Autodesk Inventor part; units mm, degrees
ref_plane "YZ Plane" through (0, 0, 0) normal (1, 0, 0) x (0, 1, 0)
ref_plane "XZ Plane" through (0, 0, 0) normal (0, 1, 0) x (-1, 0, 0)
ref_plane "XY Plane" through (0, 0, 0) normal (0, 0, 1) x (1, 0, 0)
sketch "Sketch1" plane through (0, 0, 0) normal (0, 1, 0) x (-1, 0, 0)
  circle A0 centre (0, 0) radius 4.9
  circle A1 centre (0, 0) radius 6.9
  line L0 (6.9, 8) -> (-5.9499, 8) construction
  line L1 (6.9, -8) -> (-5.9499, -8) construction
  line L2 (8, 8.15) -> (-8, 8.15)
  line L3 (-8, 8.15) -> (-8, -8.15)
  line L4 (-8, -8.15) -> (8, -8.15)
  line L5 (8, -8.15) -> (8, 8.15)
  line L6 (8, 8.15) -> (8, 10.15)
  line L7 (8, 10.15) -> (-8, 10.15)
  line L8 (-8, 10.15) -> (-8, 8.15)
  line L9 (-8, -8.15) -> (-8, -10.15)
  line L10 (-8, -10.15) -> (8, -10.15)
  line L11 (8, -10.15) -> (8, -8.15)
  point P0 (0, -8.15)
  dimension "d0" = 9.8
  dimension "d1" = 2
  dimension "d2" = 16
  dimension "d3" = 8
  dimension "d4" = 0.15
  dimension "d5" = 0.15
  dimension "d6" = 16
  dimension "d7" = 2
  dimension "d8" = 2
extrude "Extrusion1" add sketch "Sketch1" along normal blind 3 contours A1 | L5 L4 L3 L2 | L2 L8 L7 L6 | L11 L10 L9 L4
extrude "Extrusion2" add sketch "Sketch1" against normal blind 15 contours L2 L8 L7 L6 | L11 L10 L9 L4
sketch "Sketch2" plane through (-8, 3, 10.15) normal (0, 0, 1) x (1, 0, 0)
  circle A0 centre (8, -15) radius 1.65
  line L0 (16, -18) -> (0, -18)
  point P0 (8, -3)
  point P1 (8, -18)
  dimension "d13" = 3.3
  dimension "d14" = 3
extrude "Extrusion3" cut sketch "Sketch2" against normal through all
sketch "Sketch3" plane through (-8, 3, 10.15) normal (0, 0, 1) x (1, 0, 0)
  line L0 (8, -10) -> (8, -6) construction
  line L1 (9.65, -10) -> (9.65, -6)
  line L2 (6.35, -6) -> (6.35, -10)
  arc A0 (6.35, -10) -> (9.65, -10) centre (8, -10) ccw
  arc A1 (9.65, -6) -> (6.35, -6) centre (8, -6) ccw
  circle A2 centre (8, -15) radius 1.65
  point P0 (8, -3)
  point P1 (8, -8)
  dimension "d17" = 3.3
  dimension "d18" = 4
  dimension "d19" = 5
extrude "Extrusion4" cut sketch "Sketch3" against normal through all contours A0 L2 A1 L1
properties part number "ShaftSyncAdapter" material "ABS Plastic"
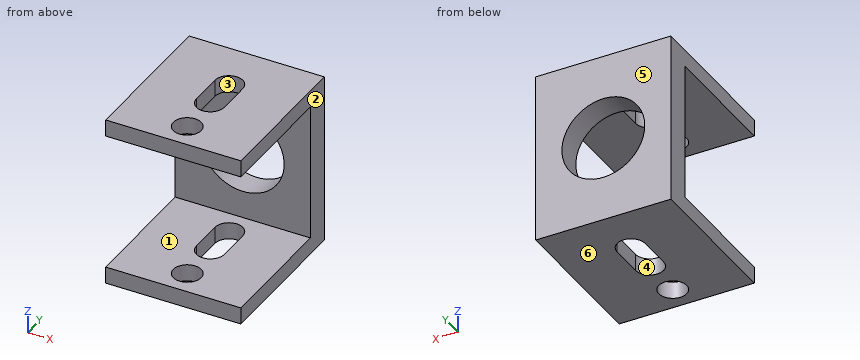
CAD build for the part. Positions are in the model's coordinates, mm. Face numbers are marked on the shaded views. A direction names the side the tool comes from. Give positions to 0.01 mm unless a question says otherwise; leave off trailing zeros. Write each loop counter-clockwise with the first axis right and the second up, starting at its lowest first coordinate (ties: lowest second). Pieces come first, ordered by that corner, then holes. Notation, with made-up numbers: (25, -23.5) - (54, -23.5) arc R21 cw to (54, -8.5) - close; hole circle Ø2 at (25, 56). An arc over 180 degrees is marked (long way). Put each result on its own line as item: value.
(1) Wall check: L1, parallel to Y at x = 0, z = 8.85; L2, parallel to Z at x = -6.75, y = -9.5; L3, parallel to Z at x = 0, y = 0.9. Give the ranges that are in metal, low to high.
Working result:
L1: -15 to -13.65, -10.35 to -8.65, -1.35 to 3
L2: -10.15 to -8.15, 8.15 to 10.15
L3: -10.15 to -4.9, 4.9 to 10.15
(2) Saw through at B-B (x = 0). List the corners of the cut face in (y, z).
Working result:
outline: (-15, -10.15) - (-13.65, -10.15) - (-13.65, -8.15) - (-15, -8.15) - close; (-15, 8.15) - (-13.65, 8.15) - (-13.65, 10.15) - (-15, 10.15) - close; (-10.35, -10.15) - (-8.65, -10.15) - (-8.65, -8.15) - (-10.35, -8.15) - close; (-10.35, 8.15) - (-8.65, 8.15) - (-8.65, 10.15) - (-10.35, 10.15) - close; (-1.35, -10.15) - (3, -10.15) - (3, -4.9) - (0, -4.9) - (0, -8.15) - (-1.35, -8.15) - close; (-1.35, 8.15) - (0, 8.15) - (0, 4.9) - (3, 4.9) - (3, 10.15) - (-1.35, 10.15) - close
(3) Tool access for the marked faces 1, 2 and 3: list every direction of +Z, -Z, +X, -X, +Y, -Y with a clear straight run to the whole face (end or side of a thin tool).
Working result:
face 1: +X, -X, -Y
face 2: +Z, -Z, +X, +Y, -Y
face 3: +Z, -Z
(4) Drop a flat-ended pin along its axis: pin 1 Ø8 at (x, z) = (1, 3.5) entering from -Y. Give the stop position or say it passes through.
Working result:
pin 1: y = 0
(5) Saw through at D-D (x = -2.75). List the corners of the cut face in (y, z).
Working result:
outline: (-15, -10.15) - (3, -10.15) - (3, -4.06) - (0, -4.06) - (0, -8.15) - (-15, -8.15) - close; (-15, 8.15) - (0, 8.15) - (0, 4.06) - (3, 4.06) - (3, 10.15) - (-15, 10.15) - close
(6) Saw through at A-A (y = -12). List the corners of the cut face in (x, z), then the cut area to 3 significant figures.
Working result:
outline: (-8, -10.15) - (-1.65, -10.15) - (-1.65, -8.15) - (-8, -8.15) - close; (-8, 8.15) - (-1.65, 8.15) - (-1.65, 10.15) - (-8, 10.15) - close; (1.65, -10.15) - (8, -10.15) - (8, -8.15) - (1.65, -8.15) - close; (1.65, 8.15) - (8, 8.15) - (8, 10.15) - (1.65, 10.15) - close
area: 50.8 mm^2
(7) Saw through at C-C (z = 0). List the corners of the cut face in (x, y).
Working result:
outline: (-8, 0) - (-4.9, 0) - (-4.9, 3) - (-8, 3) - close; (4.9, 0) - (8, 0) - (8, 3) - (4.9, 3) - close
(8) Pull direction Y, two halves, no side cores. Call the marked faces 4, 5 and 6: released by +Y, released by -Y, zero draft, split by the parting line, or undercut.
Working result:
face 4: undercut
face 5: released by +Y
face 6: zero draft
